Solid Edge part; units mm, degrees
sketch "Sketch1" plane through (0, 0, 0) normal (0, 0, 1) x (1, 0, 0)
  circle A0 centre (0, 0) radius 3.1
extrude "Protrusion1" add sketch "Sketch1" along normal blind 21
sketch "Sketch2" plane through (0, 0, 0) normal (0, 0, -1) x (1, 0, 0)
  line L0 (3.1, 3.1) -> (-3.1, 3.1)
  line L1 (-3.1, 3.1) -> (-3.1, -3.1)
  line L2 (-3.1, -3.1) -> (3.1, -3.1)
  line L3 (3.1, -3.1) -> (3.1, 3.1)
extrude "ExtrudedProtrusion_2" add sketch "Sketch2" against normal blind 1
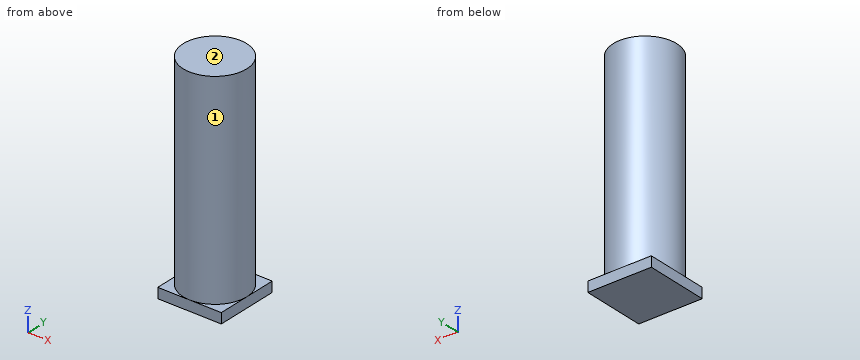
For this review, take the finished solid that the model builds, in its own axes (mm). Face numbers are marked on the shaded views. A direction names the side the tool comes from. Round coordinates to 2 decimals unless told otherwise and drop trailing zeros. Order: outer loops, then holes, each group sorted by start corner. A loop starts at its lowest first (then second) coordinate and runs counter-clockwise, first axis right, second up. Notation, with made-up numbers: (-2, -35) -> (41, -35) arc R21 cw to (41, -18) -> close; hole circle Ø5 at (-15, -14). An arc over 180 degrees is marked (long way). Use a Markdown table: item, result.
Item 1: Machinability: for the marked faces 1 and 2, which of the approach directions +Z, -Z, +X, -X, +Y, -Y give a long, thin tool a straight path to every point of the face, cutting with its end or side? Answer none if there is none.
Resolved:
| item | result |
|---|---|
| face 1 | +Z |
| face 2 | +Z, +X, -X, +Y, -Y |
Item 2: For line 1 along X through (y, z) = (-2, 3.5); line 2 along Z through (x, y) = (2.75, -2); line 3 along X through (y, z) = (-1.5, 15.5), list the stretches that pass through material, from the lowest coordinate up. Write a range as [from, to].
Resolved:
| item | result |
|---|---|
| line 1 | x = [-2.37, 2.37] |
| line 2 | z = [0, 1] |
| line 3 | x = [-2.71, 2.71] |
Item 3: Take a section at B-B (x = -1). State the section outline as (y, z) points.
Resolved:
| item | result |
|---|---|
| outline | (-3.1, 0) -> (3.1, 0) -> (3.1, 1) -> (2.93, 1) -> (2.93, 21) -> (-2.93, 21) -> (-2.93, 1) -> (-3.1, 1) -> close |
Item 4: Take a section at A-A (y = 1.25). State the section outline as (x, z) points.
Resolved:
| item | result |
|---|---|
| outline | (-3.1, 0) -> (3.1, 0) -> (3.1, 1) -> (2.84, 1) -> (2.84, 21) -> (-2.84, 21) -> (-2.84, 1) -> (-3.1, 1) -> close |
Item 5: For pin 1 (2 mm diameter, centred on x = -2.5, z = 13.5, fed in from -Y); pin 2 (1.5 mm diameter, centred on x = -1, z = 7, fed in from +Y); pin 3 (3 mm diameter, centred on x = 0.5, z = 18, fed in from -Y), all flat-tipped, find the tip position at first contact; note any pin that passes through.
Resolved:
| item | result |
|---|---|
| pin 1 | stops at y = -2.71 |
| pin 2 | stops at y = 3.09 |
| pin 3 | stops at y = -3.1 |
Item 6: Take a section at C-C (z = 16.5). State the section outline as (x, y) points, plus the area to 3 significant figures.
Resolved:
| item | result |
|---|---|
| outline | circle Ø6.2 at (0, 0) |
| area | 30.2 mm² |
